The drawing under review shows one solid part. Ordinate dimensions are in mm from its lowest x, y, z. A direction names the side the tool comes from. Coordinates: 2 decimals unless noted, no trailing zeros. Write each loop counter-clockwise with the first axis right and the second up, starting at its lowest first coordinate (ties: lowest second). Pieces come first, ordered by that corner, then holes.
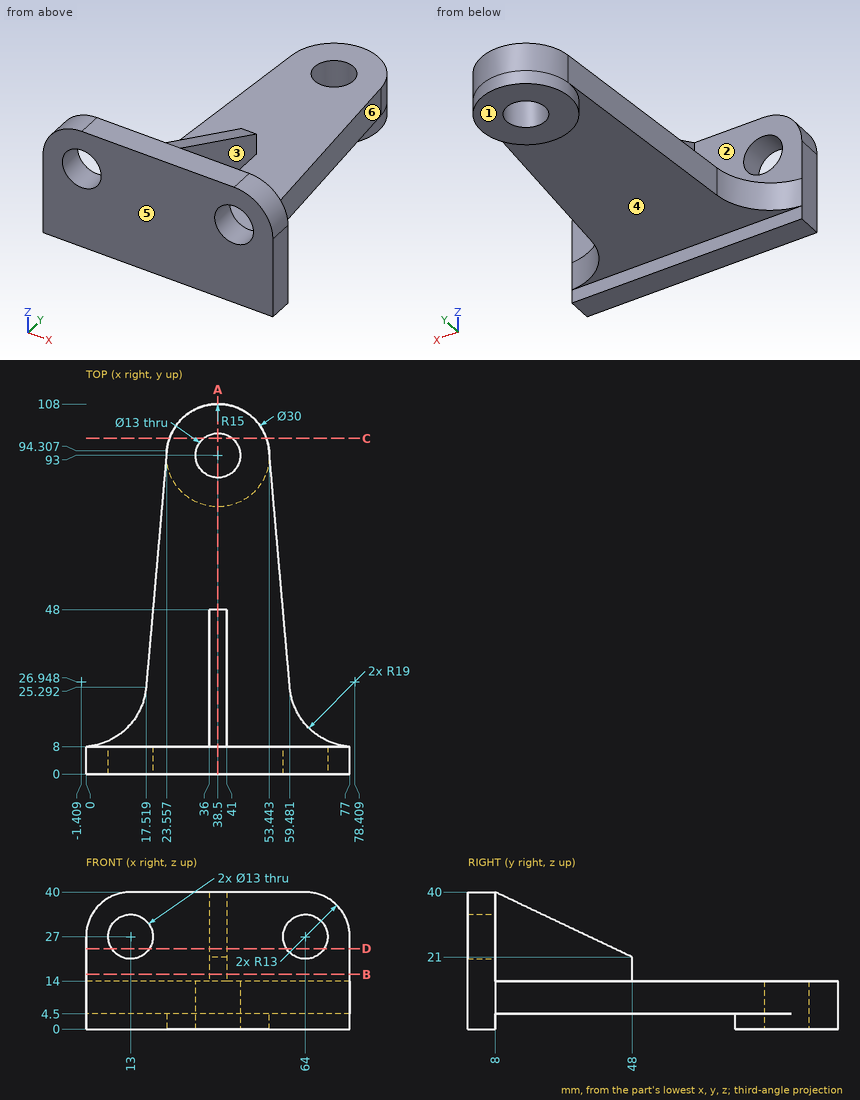
Q1. Tool access review of the marked faces 1, 2 and 3: name each direction out of +Z, -Z, +X, -X, +Y, -Y from which nothing blocks a thin tool from reaching the whole face with its end or side.
Ans:
face 1: -Z, +X, -X, +Y, -Y
face 2: +Z, -X, +Y
face 3: +Z, +X, +Y
Q2. Add section C-C (y = 98). State the section outline as (x, z) points, then the cut area to 3 significant figures.
Ans:
outline: (24.36, 0) - (34.35, 0) - (34.35, 14) - (24.36, 14) - close; (42.65, 0) - (52.64, 0) - (52.64, 14) - (42.65, 14) - close
area: 280 mm2
Q3. Add section B-B (z = 16). State the section outline as (x, y) points.
Ans:
outline: (0, 0) - (77, 0) - (77, 8) - (41, 8) - (41, 48) - (36, 48) - (36, 8) - (0, 8) - close
Q4. Clearance check with flat-ended pins moving along their axes: pin 1 Ø13 at (y, z) = (35, 26.5) entering from -X; pin 2 Ø10 at (x, y) = (20, 66) entering from +Z; pin 3 Ø6 at (x, y) = (53.5, 73) entering from -Z. State where each tip first meets the part, or that it passes through.
Ans:
pin 1: stops at x = 36
pin 2: stops at z = 14
pin 3: stops at z = 4.5
Q5. Add section A-A (x = 38.5). State the section outline as (y, z) points.
Ans:
outline: (0, 0) - (8, 0) - (8, 4.5) - (78, 4.5) - (78, 0) - (86.5, 0) - (86.5, 14) - (48, 14) - (48, 21) - (8, 40) - (0, 40) - close; (99.5, 0) - (108, 0) - (108, 14) - (99.5, 14) - close
Q6. Draft analysis for pull direction Y (two halves, no side actions). For the marked faces 4, 5 and 6, state which applies: +Y half, -Y half, draft (parallel to the pull), parting line (faces both ways), or undercut.
Ans:
face 4: undercut
face 5: -Y half
face 6: +Y half
Q7. For probe 1 along X at (y, z) = (3, 27); probe 2 along Y at (x, z) = (38.5, 4); probe 3 along Z at (x, y) = (13, 5.25), list the stretches that pass through material, from the lowest coordinate up.
Ans:
probe 1: x = 0 to 6.5, 19.5 to 57.5, 70.5 to 77
probe 2: y = 0 to 8, 78 to 86.5, 99.5 to 108
probe 3: z = 0 to 20.5, 33.5 to 40
Q8. Add section D-D (z = 23.5). State the section outline as (x, y) points.
Ans:
outline: (0, 0) - (7.52, 0) - (7.52, 8) - (0, 8) - close; (18.48, 0) - (58.52, 0) - (58.52, 8) - (41, 8) - (41, 42.74) - (36, 42.74) - (36, 8) - (18.48, 8) - close; (69.48, 0) - (77, 0) - (77, 8) - (69.48, 8) - close
